```python
from build123d import *

# Parameters (mm, degrees)
F0_R     = 6.4
F1_DEPTH = 20
F3_DEPTH = 6
F4_R     = 2
F5_DEPTH = 14


# Not quite as in the source:
# - a feature names something its author has since deleted; it is built from what else it names


with BuildPart() as f1:
    # F0 (on Top) → F1 (new body)
    with BuildSketch(Plane.XY):
        Circle(F0_R)
    extrude(amount=F1_DEPTH)

    # F2 (on face) → F3 (cut)
    with BuildSketch(Plane.XY.offset(20)):
        with BuildLine():
            Line((1.942775077, 1.875), (-1.942775077, 1.875))
            ThreePointArc((-1.942775077, 1.875), (-2.7, 0), (-1.942775077, -1.875))
            Line((-1.942775077, -1.875), (1.942775077, -1.875))
            ThreePointArc((1.942775077, -1.875), (2.7, 0), (1.942775077, 1.875))
        make_face()
    extrude(amount=-F3_DEPTH, mode=Mode.SUBTRACT)

    # F4 (on face) → F5 (cut, through all)
    with BuildSketch(Plane(origin=(0, 0, 0), x_dir=(1, 0, 0), z_dir=(0, 0, -1))):
        Circle(F4_R)
    extrude(amount=-F5_DEPTH, mode=Mode.SUBTRACT)


solid = f1.part
```
Input: part model. Units: mm. Frame: model coordinates. A direction names the side the tool comes from. Coordinates: 2 decimals unless noted, no trailing zeros. Loops run counter-clockwise (first coordinate to the right, second up) from the corner with the lowest first, then second, coordinate; pieces in that order, holes last. Notation, with made-up numbers: M 41.25,63 L 46.25,63 A16 cw 46.25,89 Z; hole C 64.25,-33 d9. An arc over 180 degrees is marked long. One line per item, written item: value.
(1) Section C-C (z = 6.75). Output: boundary loops of the cut face in (x, y).
Filled in:
outline: C 0,0 d12.8; hole C 0,0 d4
(2) Reachability of faces 1 (the flat face through (3, 0, 20)), 2 (the cylindrical face through (0, 2, 7)), 3 (the flat face through (2.4, 0, 14)) from +Z, -Z, +X, -X, +Y, -Y: full face, straight path, thin tool, end or side. Return the list, or none.
Filled in:
face 1: +Z, +X, -X, +Y, -Y
face 2: -Z
face 3: +Z
(3) Section D-D (z = 17.25). Output: boundary loops of the cut face in (x, y) (3 decimals), and give its area (3 significant figures).
Filled in:
outline: C 0,0 d12.8; hole M -1.943,-1.875 L 1.943,-1.875 A2.7 ccw 1.943,1.875 L -1.943,1.875 A2.7 ccw Z
area: 110 mm^2
(4) Pull-direction query (Y, two-part tool) for faces 4 (the flat face through (1, 2, 0)), 5 (the cylindrical face through (-5.08, -3.89, 9.86)), 6 (the flat face through (0, 1.875, 17)); classes: +Y half, -Y half, draft (parallel to the pull), parting line (faces both ways), or undercut.
Filled in:
face 4: draft
face 5: parting line
face 6: undercut
(5) Section B-B (x = 0). Output: boundary loops of the cut face in (y, z) (3 decimals).
Filled in:
outline: M -6.4,0 L -2,0 L -2,14 L -1.875,14 L -1.875,20 L -6.4,20 Z; M 1.875,14 L 2,14 L 2,0 L 6.4,0 L 6.4,20 L 1.875,20 Z
(6) Section A-A (y = 0). Output: boundary loops of the cut face in (x, z).
Filled in:
outline: M -6.4,0 L -2,0 L -2,14 L -2.7,14 L -2.7,20 L -6.4,20 Z; M 2,0 L 6.4,0 L 6.4,20 L 2.7,20 L 2.7,14 L 2,14 Z
(7) Pin query (flat end, axial travel): pin 1 (3 mm diameter, centred on x = -1, z = 15.5, fed in from -Y); pin 2 (4 mm diameter, centred on y = -3, z = 10, fed in from -X). Return the tip coordinate at first contact, or that it passes through.
Filled in:
pin 1: y = -6.4
pin 2: x = -6.32
(8) Line query: line 1 along Y through (x, z) = (0, 10.5); line 2 along X through (y, z) = (-1.5, 14.25) (3 decimals); line 3 along Y through (x, z) = (-0.5, 9.75). Output: solid intervals per line, ascending. Write a range as from..to.
Filled in:
line 1: -6.4..-2, 2..6.4
line 2: -6.222..-2.245, 2.245..6.222
line 3: -6.38..-1.94, 1.94..6.38
